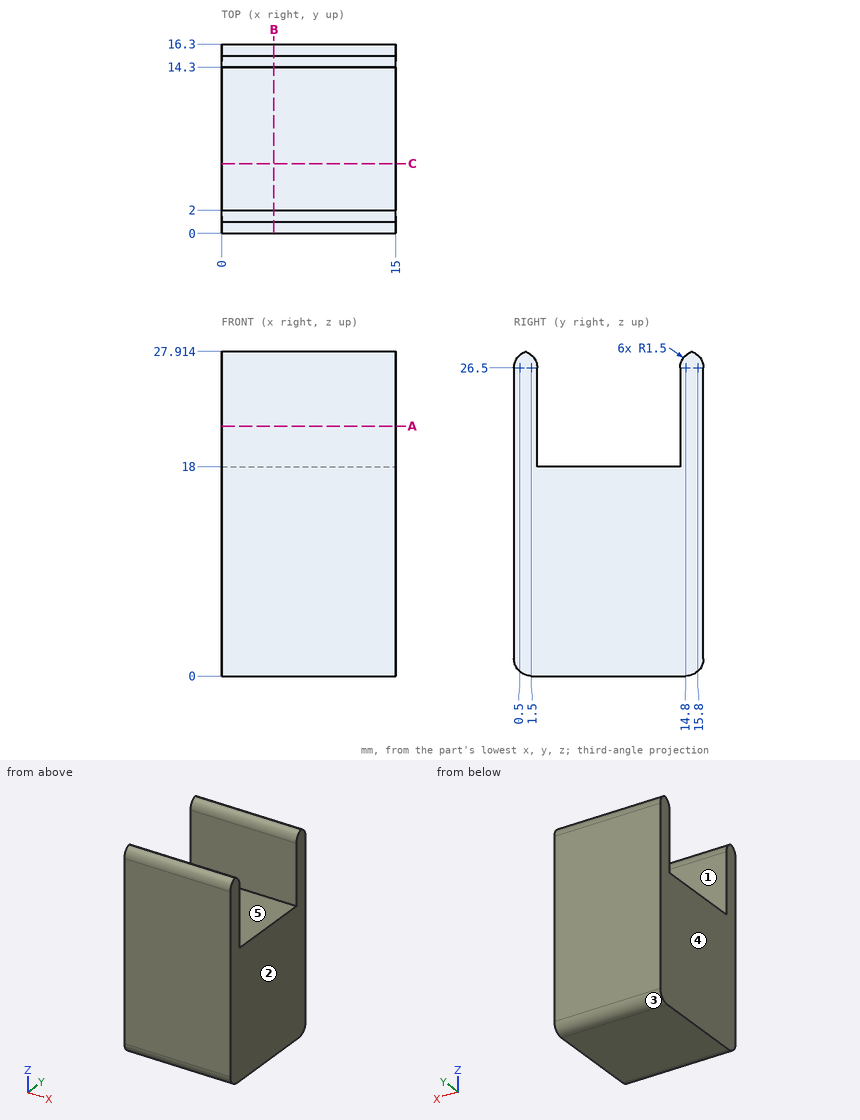
Design review of the part shown in the three views and the two pictorial views. Dimensions are in mm from the part's minimum x, y and z. A direction names the side the tool comes from. Give positions to 0.01 mm unless a question says otherwise; leave off trailing zeros. Write each loop counter-clockwise with the first axis right and the second up, starting at its lowest first coordinate (ties: lowest second). Pieces come first, ordered by that corner, then holes. Notation, with made-up numbers: M 39,59 L 86,59 A20 ccw 86,81 Z; hole C 88,-4 d4. An arc over 180 degrees is marked long. Answer in a Markdown table with one row per item.
Item 1: Add section B-B on x = 4.5. Give the boundary of the cut face in (y, z), plus the area to 3 significant figures.
Check sheet entries:
| item | result |
|---|---|
| outline | M 0,1.5 A1.5 ccw 1.5,0 L 14.8,0 A1.5 ccw 16.3,1.5 L 16.3,26.5 A1.5 ccw 15.3,27.91 A1.5 ccw 14.3,26.5 L 14.3,18 L 2,18 L 2,26.5 A1.5 ccw 1,27.91 A1.5 ccw 0,26.5 Z |
| area | 331 mm2 |
Item 2: Draft analysis for pull direction Y (two halves, no side actions). For the marked faces 3, 4 and 5, state which applies: +Y half, -Y half, draft (parallel to the pull), parting line (faces both ways), or undercut.
Check sheet entries:
| item | result |
|---|---|
| face 3 | +Y half |
| face 4 | draft |
| face 5 | undercut |
Item 3: Add section A-A on z = 21.5. Give the boundary of the cut face in (x, y), plus the area to 3 significant figures.
Check sheet entries:
| item | result |
|---|---|
| outline | M 0,0 L 15,0 L 15,2 L 0,2 Z; M 0,14.3 L 15,14.3 L 15,16.3 L 0,16.3 Z |
| area | 60.0 mm2 |
Item 4: Add section C-C on y = 6. Give the boundary of the cut face in (x, z), plus the area to 3 significant figures.
Check sheet entries:
| item | result |
|---|---|
| outline | M 0,0 L 15,0 L 15,18 L 0,18 Z |
| area | 270 mm2 |
Item 5: For P1, Ø5, axis at x = 12, y = 6.5, coming from the +Z side, flat-tipped, find the tip position at first contact; note if it passes through.
Check sheet entries:
| item | result |
|---|---|
| P1 | z = 18 |
Item 6: For line 1 along Y through (x, z) = (5.5, 25); line 2 along Z through (x, y) = (4.25, 11.75); line 3 along Z through (x, y) = (6.5, 15.5), list the stretches that pass through material, from the lowest coordinate up.
Check sheet entries:
| item | result |
|---|---|
| line 1 | 0 to 2, 14.3 to 16.3 |
| line 2 | 0 to 18 |
| line 3 | 0.17 to 27.83 |
Item 7: Tool access review of the marked faces 1 and 2: name each direction out of +Z, -Z, +X, -X, +Y, -Y from which nothing blocks a thin tool from reaching the whole face with its end or side.
Check sheet entries:
| item | result |
|---|---|
| face 1 | +Z, +X, -X |
| face 2 | +Z, -Z, +X, +Y, -Y |
